CAD build for the part. Positions are in the model's coordinates, mm. Face numbers are marked on the shaded views. Coordinates: 2 decimals unless noted, no trailing zeros. Order: outer loops, then holes, each group sorted by start corner. A loop starts at its lowest first (then second) coordinate and runs counter-clockwise, first axis right, second up. Notation, with made-up numbers: (-10, -29.5) - (8, -29.5) arc R37 ccw to (8, 6.5) - close; hole circle Ø6 at (83, 35.25). An arc over 180 degrees is marked (long way). Use one line per item in the form item = value.
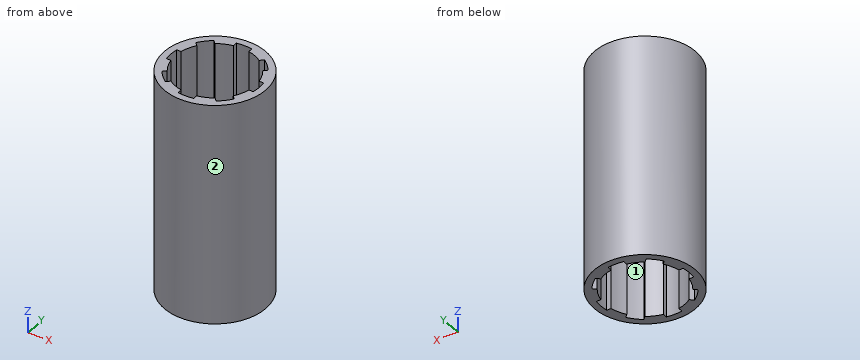
```python
from build123d import *

# Parameters (mm, degrees)
SKETCH_1_R      = 23
SKETCH_1_R_2    = 20
EXTRUDE_1_DEPTH = 100
EXTRUDE_START   = -100
EXTRUDE_2_DEPTH = 100


with BuildPart() as part:
    # 草图1 → 凸台-拉伸1 (new body)
    with BuildSketch(Plane.XY):
        Circle(SKETCH_1_R)
        Circle(SKETCH_1_R_2, mode=Mode.SUBTRACT)
    extrude(amount=EXTRUDE_1_DEPTH)

    # 草图2 → 凸台-拉伸2 (add)
    with BuildSketch(Plane.XY.offset(100).offset(EXTRUDE_START)):
        with BuildLine():
            Line((-14.959864723, 10.010117255), (-16.39877405, 11.449026581))
            ThreePointArc((-16.39877405, 11.449026581), (-18.47759065, 7.653668647), (-19.691368668, 3.5))
            Line((-19.691368668, 3.5), (-17.656443583, 3.5))
            ThreePointArc((-17.656443583, 3.5), (-16.629831585, 6.888301783), (-14.959864723, 10.010117255))
        make_face()
        with BuildLine():
            Line((-3.5, 17.656443583), (-3.5, 19.691368668))
            ThreePointArc((-3.5, 19.691368668), (-7.653668647, 18.47759065), (-11.449026581, 16.39877405))
            Line((-11.449026581, 16.39877405), (-10.010117255, 14.959864723))
            ThreePointArc((-10.010117255, 14.959864723), (-6.888301783, 16.629831585), (-3.5, 17.656443583))
        make_face()
        with BuildLine():
            Line((10.010117255, 14.959864723), (11.449026581, 16.39877405))
            ThreePointArc((11.449026581, 16.39877405), (7.653668647, 18.47759065), (3.5, 19.691368668))
            Line((3.5, 19.691368668), (3.5, 17.656443583))
            ThreePointArc((3.5, 17.656443583), (6.888301783, 16.629831585), (10.010117255, 14.959864723))
        make_face()
        with BuildLine():
            ThreePointArc((19.691368668, 3.5), (18.47759065, 7.653668647), (16.39877405, 11.449026581))
            Line((16.39877405, 11.449026581), (14.959864723, 10.010117255))
            ThreePointArc((14.959864723, 10.010117255), (16.629831585, 6.888301783), (17.656443583, 3.5))
            Line((17.656443583, 3.5), (19.691368668, 3.5))
        make_face()
        with BuildLine():
            ThreePointArc((16.39877405, -11.449026581), (18.47759065, -7.653668647), (19.691368668, -3.5))
            Line((19.691368668, -3.5), (17.656443583, -3.5))
            ThreePointArc((17.656443583, -3.5), (16.629831585, -6.888301783), (14.959864723, -10.010117255))
            Line((14.959864723, -10.010117255), (16.39877405, -11.449026581))
        make_face()
        with BuildLine():
            ThreePointArc((3.5, -19.691368668), (7.653668647, -18.47759065), (11.449026581, -16.39877405))
            Line((11.449026581, -16.39877405), (10.010117255, -14.959864723))
            ThreePointArc((10.010117255, -14.959864723), (6.888301783, -16.629831585), (3.5, -17.656443583))
            Line((3.5, -17.656443583), (3.5, -19.691368668))
        make_face()
        with BuildLine():
            Line((-10.010117255, -14.959864723), (-11.449026581, -16.39877405))
            ThreePointArc((-11.449026581, -16.39877405), (-7.653668647, -18.47759065), (-3.5, -19.691368668))
            Line((-3.5, -19.691368668), (-3.5, -17.656443583))
            ThreePointArc((-3.5, -17.656443583), (-6.888301783, -16.629831585), (-10.010117255, -14.959864723))
        make_face()
        with BuildLine():
            Line((-17.656443583, -3.5), (-19.691368668, -3.5))
            ThreePointArc((-19.691368668, -3.5), (-18.47759065, -7.653668647), (-16.39877405, -11.449026581))
            Line((-16.39877405, -11.449026581), (-14.959864723, -10.010117255))
            ThreePointArc((-14.959864723, -10.010117255), (-16.629831585, -6.888301783), (-17.656443583, -3.5))
        make_face()
    extrude(amount=EXTRUDE_2_DEPTH)


solid = part.part
```
Item 1: Two-plate mould, pull along X, no slides. Class the marked faces 1 and 2: +X half, -X half, draft (parallel to the pull), parting line (faces both ways), or undercut.
Derived:
face_1 = undercut
face_2 = parting line
Item 2: Cut at C-C, the plane y = 6.5. Write the cut outline in (x, z).
Derived:
outline = (-22.06, 0) - (-16.79, 0) - (-16.79, 100) - (-22.06, 100) - close; (16.79, 0) - (22.06, 0) - (22.06, 100) - (16.79, 100) - close
Item 3: Cut at A-A, the plane x = 0. Write the cut outline in (y, z).
Derived:
outline = (-23, 0) - (-20, 0) - (-20, 100) - (-23, 100) - close; (20, 0) - (23, 0) - (23, 100) - (20, 100) - close
Item 4: Drill centre lines: line 1 (X direction, y = -16, z = 43); line 2 (X direction, y = 0.5, z = 20). Where is each one in solid material? Low to high. Write a range as [from, to].
Derived:
line_1 = [-16.52, -12], [-11.05, -8.25], [8.25, 11.05], [12, 16.52]
line_2 = [-22.99, -19.99], [19.99, 22.99]
Item 5: Drop flat-ended pins along their axis: pin 1 (4 mm diameter, centred on y = 1, z = 25.5, fed in from -X); pin 2 (2 mm diameter, centred on y = 14.5, z = 72.5, fed in from -X); pin 3 (10 mm diameter, centred on x = -3.5, z = 85, fed in from -Y); pin 4 (0.6 mm diameter, centred on x = -18.5, z = 69.5, fed in from +Y). Give the stop position or say it passes through.
Derived:
pin_1 = -23
pin_2 = -18.62
pin_3 = -23
pin_4 = 14.06
